Source: CAD feature listing. Evaluate the final solid. Frame: model axes, mm. A direction names the side the tool comes from. Coordinates: 2 decimals unless noted, no trailing zeros. Loops run counter-clockwise (first coordinate to the right, second up) from the corner with the lowest first, then second, coordinate; pieces in that order, holes last. Notation, with made-up numbers: M -36.5,1.5 L -1.5,1.5 A23 ccw -1.5,35.5 Z; hole C -25.75,63 d2. An arc over 180 degrees is marked long. One line per question, with ' | ' between items. Start each with the question number.
1. Section query B-B, the plane z = 23. Output: boundary loops of the cut face in (x, y).
2. Pin query (flat end, axial travel): P1, Ø10, axis at y = -5.5, z = 23, coming from the -X side; P2, Ø10, axis at y = -12.7, z = 24.85, coming from the +X side; P3, Ø5, axis at x = -26, y = -17.5, coming from the +Z side; P4, Ø4, axis at y = -5, z = 9, coming from the -X side. Return the tip coordinate at first contact, or that it passes through.
3. Access query for faces 1 (the flat face through (20.4, -6.9, 12.7)), 2 (the cylindrical face through (-44.804, -12.896, 6.439)), 3 (the flat face through (-27, -15, 12.7)). Directions: +Z, -Z, +X, -X, +Y, -Y. A direction counts if a zero-diameter tool reaches every point of the face in a straight line with its end or side. Return the directions, or none.
4. Section query D-D, the plane y = -5.5. Output: boundary loops of the cut face in (x, z).
5. Ray query, probe 1 along Z at (x, y) = (26, -21.5); probe 2 along Z at (x, y) = (-8.5, -12.7); probe 3 along Z at (x, y) = (-10.5, -7.25). Return the intervals inside material, ascending.
6. Mould query, pull axis X, two halves, no side actions, for faces 4 (the flat face through (-8, -13, 0)), 5 (the cylindrical face through (12.39, -16.564, 6.439)), 6 (the cylindrical face through (28.01, -4.61, 6.44)), 7 (the cylindrical face through (-34.75, -18.9, 6.44)). Classes: pulls with the +X half, pulls with the -X half, needs draft (parallel to the pull), parting line crosses it, or undercut.
7. Section query C-C, the plane x = -17.5. Output: boundary loops of the cut face in (y, z), and give its area (3 significant figures).
8. Section query A-A, the plane y = -12.7. Output: boundary loops of the cut face in (x, z).
```python
from build123d import *

# Parameters (mm, degrees)
F1_DEPTH = 25.4
F2_R     = 6.35
F3_DEPTH = 12.701
F4_R     = 6.35
F5_DEPTH = 50.801
F7_DEPTH = 12.701
F9_DEPTH = 12.701


with BuildPart() as f1:
    # F0 (on Front) → F1 (new body)
    with BuildSketch(Plane.XZ):
        Polygon((-20.6712735461, 12.7), (-46.0712735461, 12.7), (-46.0712735461, 0), (30.1287264539, 0), (30.1287264539, 12.7), (4.7287264539, 12.7), (4.7287264539, 44.45), (-20.6712735461, 44.45), align=None)
    extrude(amount=F1_DEPTH)

    # F2 (on face) → F3 (cut, through all)
    with BuildSketch(Plane.XY.offset(12.7)):
        with Locations((17.4287264539, -12.7)):
            Circle(F2_R)
        with Locations((-33.3712735461, -12.7)):
            Circle(F2_R)
    extrude(amount=-F3_DEPTH, mode=Mode.SUBTRACT)

    # F4 (on face) → F5 (cut, through all)
    with BuildSketch(Plane.YZ.offset(4.7287264539)):
        with Locations((-12.7, 24.8512161426)):
            Circle(F4_R)
        with BuildLine():
            ThreePointArc((-25.4, 31.75), (-12.7, 39.3040089077), (0, 31.75))
            Line((0, 31.75), (0, 44.45))
            Line((0, 44.45), (-25.4, 44.45))
            Line((-25.4, 44.45), (-25.4, 31.75))
        make_face()
    extrude(amount=-F5_DEPTH, mode=Mode.SUBTRACT)

    # F6 (on face) → F7 (cut, through all)
    with BuildSketch(Plane.XY.offset(12.7)):
        with BuildLine():
            ThreePointArc((-39.7212735461, -25.4), (-44.8051245149, -12.7), (-39.7212735461, 0))
            Line((-39.7212735461, 0), (-46.0712735461, 0))
            Line((-46.0712735461, 0), (-46.0712735461, -25.4))
            Line((-46.0712735461, -25.4), (-39.7212735461, -25.4))
        make_face()
    extrude(amount=-F7_DEPTH, mode=Mode.SUBTRACT)

    # F8 (on face) → F9 (cut, through all)
    with BuildSketch(Plane.XY.offset(12.7)):
        with BuildLine():
            ThreePointArc((23.7787264539, 0), (28.0557438818, -4.6825889157), (30.1287264539, -10.6761071051))
            Line((30.1287264539, -10.6761071051), (30.1287264539, 0))
            Line((30.1287264539, 0), (23.7787264539, 0))
        make_face()
        with BuildLine():
            ThreePointArc((30.1287264539, -14.7238928949), (28.0557438818, -20.7174110843), (23.7787264539, -25.4))
            Line((23.7787264539, -25.4), (30.1287264539, -25.4))
            Line((30.1287264539, -25.4), (30.1287264539, -14.7238928949))
        make_face()
    extrude(amount=-F9_DEPTH, mode=Mode.SUBTRACT)


solid = f1.part
```
Taken from the geometry:
1) outline: M -20.67,-25.4 L 4.73,-25.4 L 4.73,-18.77 L -20.67,-18.77 Z; M -20.67,-6.63 L 4.73,-6.63 L 4.73,0 L -20.67,0 Z
2) P1: x = -20.67 | P2: through | P3: z = 12.7 | P4: x = -43.9
3) face 1: +Z, +X, +Y, -Y | face 2: +Z, -Z, -X | face 3: +Z, -X, +Y, -Y
4) outline: M -43.34,0 L 28.51,0 L 28.51,12.7 L 4.73,12.7 L 4.73,37.38 L -20.67,37.38 L -20.67,12.7 L -43.34,12.7 Z
5) probe 1: 0 to 12.7 | probe 2: 0 to 18.5, 31.2 to 39.3 | probe 3: 0 to 21.59, 28.11 to 38.24
6) face 4: needs draft | face 5: undercut | face 6: pulls with the +X half | face 7: undercut
7) outline: M -25.4,0 L 0,0 L 0,31.75 A14.45 ccw -25.4,31.75 Z; hole C -12.7,24.85 d12.7 | area: 816 mm^2
8) outline: M -44.81,0 L -39.72,0 L -39.72,12.7 L -44.81,12.7 Z; M -27.02,0 L 11.08,0 L 11.08,12.7 L 4.73,12.7 L 4.73,18.5 L -20.67,18.5 L -20.67,12.7 L -27.02,12.7 Z; M -20.67,31.2 L 4.73,31.2 L 4.73,39.3 L -20.67,39.3 Z; M 23.78,0 L 30.13,0 L 30.13,12.7 L 23.78,12.7 Z
